```python
from build123d import *

# Parameters (mm, degrees)
F0_W     = 60
F0_H     = 9
F1_DEPTH = 6.6
F2_W     = 48.626702
F2_H     = 3.214986
F2_R     = 0.929944
F3_DEPTH = 1
F4_W     = 3.7
F4_H     = 1.2
F5_DEPTH = 21.6


with BuildPart() as f1:
    # F0 (on Top) → F1 (new body)
    with BuildSketch(Plane.XY):
        Rectangle(F0_W, F0_H)
    extrude(amount=-F1_DEPTH)

    # F2 (on face) → F3 (cut)
    with BuildSketch(Plane(origin=(0, 0, -6.6), x_dir=(1, 0, 0), z_dir=(0, 0, -1))):
        Rectangle(F2_W, F2_H)
        with Locations((-27.945412, 0)):
            Circle(F2_R)
        with Locations((27.945412, 0)):
            Circle(F2_R)
    extrude(amount=-F3_DEPTH, mode=Mode.SUBTRACT)

    # F4 (on face) → F5 (join)
    with BuildSketch(Plane.XY):
        Rectangle(F4_W, F4_H)
    extrude(amount=-F5_DEPTH)


solid = f1.part
```
CAD build for the part. Positions are in the model's coordinates, mm. A direction names the side the tool comes from. Give positions to 0.01 mm unless a question says otherwise; leave off trailing zeros. Order: outer loops, then holes, each group sorted by start corner. A loop starts at its lowest first (then second) coordinate and runs counter-clockwise, first axis right, second up.
(1) Saw through at B-B, the plane y = 0. Give the cut face in (x, z), then the cut area to 3 significant figures.
(2) Saw through at C-C, the plane z = -14.75. Give the cut face in (x, y).
(3) Mould opens along X. For faces 1 (the flat face through (-24.313, 0, -6)), 2 (the flat face through (30, 0, -3)), 3 (the flat face through (0, 4.5, -3)) say: released by +X, released by -X, zero draft, split by the parting line, or undercut.
(4) Flat gauge pins, fed straight in: pin 1 (1 mm diameter, centred on y = -1, z = -12.5, fed in from -X); pin 2 (1.8 mm diameter, centred on x = -1, z = -15.5, fed in from +Y); pin 3 (3 mm diameter, centred on x = -23, y = 2.5, fed in from -Z). Where does each tip first touch, or does it go through?
(5) Drill centre lines: L1, parallel to X at y = 0, z = -6.05; L2, parallel to Y at x = -1.5, z = -5.75; L3, parallel to Y at x = -0.5, z = -14. Where is each one in solid material? Low to high.
(6) Saw through at A-A, the plane x = -0.5. Give the cut face in (y, z), then the cut area to 3 significant figures.
(7) Saw through at D-D, the plane x = 19. Give the cut face in (y, z).
(8) Tool access for faces 4 (the cylindrical face through (-28.874, -0.041, -6.107)), 5 (the flat face through (-30, 0, -3)): list every direction of +Z, -Z, +X, -X, +Y, -Y with a clear straight run to the whole face (end or side of a thin tool).
Results found:
1. outline: (-30, -6.6) - (-28.88, -6.6) - (-28.88, -5.6) - (-27.02, -5.6) - (-27.02, -6.6) - (-24.31, -6.6) - (-24.31, -5.6) - (-1.85, -5.6) - (-1.85, -21.6) - (1.85, -21.6) - (1.85, -5.6) - (24.31, -5.6) - (24.31, -6.6) - (27.02, -6.6) - (27.02, -5.6) - (28.88, -5.6) - (28.88, -6.6) - (30, -6.6) - (30, 0) - (-30, 0) - close
1. area: 403 mm2
2. outline: (-1.85, -0.6) - (1.85, -0.6) - (1.85, 0.6) - (-1.85, 0.6) - close
3. face 1: undercut
3. face 2: released by +X
3. face 3: zero draft
4. pin 1: stops at x = -1.85
4. pin 2: stops at y = 0.6
4. pin 3: stops at z = -6.6
5. L1: x = -30 to -28.88, -27.02 to -24.31, -1.85 to 1.85, 24.31 to 27.02, 28.88 to 30
5. L2: y = -4.5 to -1.61, -0.6 to 0.6, 1.61 to 4.5
5. L3: y = -0.6 to 0.6
6. outline: (-4.5, -6.6) - (-1.61, -6.6) - (-1.61, -5.6) - (-0.6, -5.6) - (-0.6, -21.6) - (0.6, -21.6) - (0.6, -5.6) - (1.61, -5.6) - (1.61, -6.6) - (4.5, -6.6) - (4.5, 0) - (-4.5, 0) - close
6. area: 75.4 mm2
7. outline: (-4.5, -6.6) - (-1.61, -6.6) - (-1.61, -5.6) - (1.61, -5.6) - (1.61, -6.6) - (4.5, -6.6) - (4.5, 0) - (-4.5, 0) - close
8. face 4: -Z
8. face 5: +Z, -Z, -X, +Y, -Y
